from build123d import *

# Parameters (mm, degrees)
F1_DEPTH = 50
F3_DEPTH = 45
F4_R     = 10
F5_DEPTH = 10
F6_R     = 8
F7_DEPTH = 12
F9_DEPTH = 25
F10_R    = 2


with BuildPart() as f1:
    # F0 (on Front) → F1 (new body, symmetric)
    with BuildSketch(Plane.XZ):
        with BuildLine():
            ThreePointArc((-75, -15), (-73.535534, -18.535534), (-70, -20))
            Line((-70, -20), (70, -20))
            ThreePointArc((70, -20), (73.535534, -18.535534), (75, -15))
            Line((75, -15), (75, 15))
            ThreePointArc((75, 15), (73.535534, 18.535534), (70, 20))
            Line((70, 20), (-70, 20))
            ThreePointArc((-70, 20), (-73.535534, 18.535534), (-75, 15))
            Line((-75, 15), (-75, -15))
        make_face()
        with BuildLine():
            Line((73, 15), (73, -15))
            ThreePointArc((73, -15), (72.12132, -17.12132), (70, -18))
            Line((70, -18), (-70, -18))
            ThreePointArc((-70, -18), (-72.12132, -17.12132), (-73, -15))
            Line((-73, -15), (-73, 15))
            ThreePointArc((-73, 15), (-72.12132, 17.12132), (-70, 18))
            Line((-70, 18), (70, 18))
            ThreePointArc((70, 18), (72.12132, 17.12132), (73, 15))
        make_face(mode=Mode.SUBTRACT)
    extrude(amount=F1_DEPTH, both=True)

    # F2 (on Front) → F3 (join, symmetric)
    with BuildSketch(Plane.XZ):
        with BuildLine():
            Line((-73, 15), (-73, -15))
            ThreePointArc((-73, -15), (-72.12132, -17.12132), (-70, -18))
            Line((-70, -18), (70, -18))
            ThreePointArc((70, -18), (72.12132, -17.12132), (73, -15))
            Line((73, -15), (73, 15))
            ThreePointArc((73, 15), (72.12132, 17.12132), (70, 18))
            Line((70, 18), (-70, 18))
            ThreePointArc((-70, 18), (-72.12132, 17.12132), (-73, 15))
        make_face()
    extrude(amount=F3_DEPTH, both=True)

    # F4 (on face) → F5 (cut)
    with BuildSketch(Plane.XZ.offset(45)):
        with Locations((-35, 0)):
            Circle(F4_R)
        with Locations((-5, 0)):
            Circle(F4_R)
    extrude(amount=-F5_DEPTH, mode=Mode.SUBTRACT)

    # F6 (on face) → F7 (join)
    with BuildSketch(Plane.XZ.offset(35)):
        with Locations((-5, 0)):
            Circle(F6_R)
        with Locations((-35, 0)):
            Circle(F6_R)
    extrude(amount=F7_DEPTH)

    # F8 (on face) → F9 (cut)
    with BuildSketch(Plane.XZ.offset(47)):
        with BuildLine():
            Line((-38.971294, -1.499725), (-37.598235, -1.499725))
            ThreePointArc((-37.598235, -1.499725), (-37.120455, -2.122186), (-36.497605, -2.599457))
            Line((-36.497605, -2.599457), (-36.497605, -3.91527))
            Line((-36.497605, -3.91527), (-36.497605, -4.08473))
            ThreePointArc((-36.497605, -4.08473), (-34.985556, -5.49993), (-33.501041, -4.055874))
            Line((-33.501041, -4.055874), (-33.501041, -3.944126))
            Line((-33.501041, -3.944126), (-33.501041, -2.598677))
            ThreePointArc((-33.501041, -2.598677), (-32.878992, -2.121633), (-32.401765, -1.499725))
            Line((-32.401765, -1.499725), (-31.028708, -1.499725))
            Line((-31.028708, -1.499725), (-30.971292, -1.499725))
            ThreePointArc((-30.971292, -1.499725), (-29.500069, 0.01438), (-31.000052, 1.5))
            Line((-31.000052, 1.5), (-32.401896, 1.499952))
            ThreePointArc((-32.401896, 1.499952), (-35.000103, 3), (-37.598207, 1.499773))
            Line((-37.598207, 1.499773), (-38.971294, 1.499725))
            ThreePointArc((-38.971294, 1.499725), (-40.5, 0), (-38.971294, -1.499725))
        make_face()
        with BuildLine():
            Line((-36.497605, -4.08473), (-36.497605, -3.91527))
            ThreePointArc((-36.497605, -3.91527), (-36.5, -4), (-36.497605, -4.08473))
        make_face()
        with BuildLine():
            Line((-33.501041, -3.944126), (-33.501041, -4.055874))
            ThreePointArc((-33.501041, -4.055874), (-33.5, -4), (-33.501041, -3.944126))
        make_face()
        with BuildLine():
            ThreePointArc((-31.028708, -1.499725), (-31, -1.5), (-30.971292, -1.499725))
            Line((-30.971292, -1.499725), (-31.028708, -1.499725))
        make_face()
    extrude(amount=-F9_DEPTH, mode=Mode.SUBTRACT)

    # F10
    f10_edges = [f1.edges().sort_by_distance(p)[0] for p in [
        (-43, -47, 0),
    ]]
    fillet(f10_edges, radius=F10_R)


solid = f1.part
Can you work these out from the model? Positions are in its coordinate system, mm. A direction names the side the tool comes from. Coordinates: 2 decimals unless noted, no trailing zeros. Write each loop counter-clockwise with the first axis right and the second up, starting at its lowest first coordinate (ties: lowest second). Pieces come first, ordered by that corner, then holes. Notation, with made-up numbers: (-10, 13) -> (16, 13) arc R20 ccw to (16, 41) -> close; hole circle Ø11 at (-26, 3). An arc over 180 degrees is marked (long way). Write item = value, one per line.
(1) On a 3-axis mill with a long thin cutter (end or side, diameter ignored), from which of +Z, -Z, +X, -X, +Y, -Y can I reach the whole of each face in a straight line? I mean faces 1 (the face through (72.1, 47.46, 17.14)), 2 (the face through (-75, -1, 0)), 3 (the face through (-5, -47, 0)). Say none if no direction works.
Verdict:
face_1 = +Y
face_2 = +Z, -Z, -X, +Y, -Y
face_3 = -Y
(2) Imagine slicing it at A-A (x = -35). Please give me the cut outline in (y, z).
Verdict:
outline = (-50, -20) -> (50, -20) -> (50, -18) -> (45, -18) -> (45, 18) -> (50, 18) -> (50, 20) -> (-50, 20) -> (-50, 18) -> (-45, 18) -> (-45, 10) -> (-35, 10) -> (-35, 8) -> (-45, 8) arc R2 ccw to (-47, 6) -> (-47, 3) -> (-22, 3) -> (-22, -5.5) -> (-47, -5.5) -> (-47, -6) arc R2 ccw to (-45, -8) -> (-35, -8) -> (-35, -10) -> (-45, -10) -> (-45, -18) -> (-50, -18) -> close
(3) Imagine slicing it at D-D (x = -5). Please give me the cut outline in (y, z).
Verdict:
outline = (-50, -20) -> (50, -20) -> (50, -18) -> (45, -18) -> (45, 18) -> (50, 18) -> (50, 20) -> (-50, 20) -> (-50, 18) -> (-45, 18) -> (-45, 10) -> (-35, 10) -> (-35, 8) -> (-47, 8) -> (-47, -8) -> (-35, -8) -> (-35, -10) -> (-45, -10) -> (-45, -18) -> (-50, -18) -> close
(4) Thinking about a two-plate mould opening in Z: for faces 4 (the face through (0, 50, -19)), 5 (the face through (-73, -1, 19)), 6 (the face through (-1, -45, 12)), which applies, +Z half, -Z half, draft (parallel to the pull), parting line (faces both ways), or undercut?
Verdict:
face_4 = draft
face_5 = +Z half
face_6 = undercut
(5) If I drill on probe 1 along Z at (x, y) = (-5, -39.5); probe 2 along Z at (x, y) = (-35, -42.5); probe 3 along Y at (x, z) = (51, 10.5), over which ranges is the centre line in solid material (lowest first)?
Verdict:
probe_1 = -20 to -10, -8 to 8, 10 to 20
probe_2 = -20 to -10, -8 to -5.5, 3 to 8, 10 to 20
probe_3 = -45 to 45
(6) Imagine slicing it at C-C (x = -56). Please give me the cut outline in (y, z).
Verdict:
outline = (-50, -20) -> (50, -20) -> (50, -18) -> (45, -18) -> (45, 18) -> (50, 18) -> (50, 20) -> (-50, 20) -> (-50, 18) -> (-45, 18) -> (-45, -18) -> (-50, -18) -> close
(7) For pin 1 (8 mm diameter, centred on x = -6.5, z = -1.5, fed in from -Y); pin 2 (10 mm diameter, centred on x = -42, z = -2, fed in from +Y), each with a flat end and sliding along its axis, tell me the tip position at first contact or that it passes through.
Verdict:
pin_1 = -47
pin_2 = 45
